from build123d import *

# Parameters (mm, degrees)
SKETCH1_R           = 17.5
BOSS_EXTRUDE1_DEPTH = 150
CUT_EXTRUDE1_START  = 30
CUT_EXTRUDE1_DEPTH  = 30
SKETCH4_W           = 1.6
SKETCH4_H           = 1


with BuildPart() as part:
    # Sketch1 → Boss-Extrude1 (new body)
    with BuildSketch(Plane.XY):
        Circle(SKETCH1_R)
    extrude(amount=BOSS_EXTRUDE1_DEPTH)

    # Sketch3 → Cut-Extrude1 (cut)
    with BuildSketch(Plane.XY.offset(CUT_EXTRUDE1_START)):
        with BuildLine():
            Line((-5, 16.770509831), (-5, 11.770509831))
            Line((-5, 11.770509831), (5, 11.770509831))
            Line((5, 11.770509831), (5, 16.770509831))
            ThreePointArc((5, 16.770509831), (0, 17.5), (-5, 16.770509831))
        make_face()
        with BuildLine():
            Line((16.770509831, 5), (11.770509831, 5))
            Line((11.770509831, 5), (11.770509831, -5))
            Line((11.770509831, -5), (16.770509831, -5))
            ThreePointArc((16.770509831, -5), (17.5, 0), (16.770509831, 5))
        make_face()
    extrude(amount=CUT_EXTRUDE1_DEPTH, mode=Mode.SUBTRACT)

    # Sketch4 → Cut-Revolve1 (revolve, cut)
    with BuildSketch(Plane(origin=(0, 0, 0), x_dir=(0, 0, -1), z_dir=(1, 0, 0)), mode=Mode.PRIVATE) as cut_revolve1_sk:
        with Locations((-29.2, 17)):
            Rectangle(SKETCH4_W, SKETCH4_H)
    revolve(cut_revolve1_sk.sketch.rotate(Axis((0, 0, 0), (0, 0, 1)), 90), axis=Axis((0, 0, 0), (0, 0, 1)), mode=Mode.SUBTRACT)


solid = part.part
Geometry: final body of the model. Coordinates: model frame, mm. A direction names the side the tool comes from. Give positions to 0.01 mm unless a question says otherwise; leave off trailing zeros. Write each loop counter-clockwise with the first axis right and the second up, starting at its lowest first coordinate (ties: lowest second). Pieces come first, ordered by that corner, then holes. Notation, with made-up numbers: (9.25, 30.25) -> (22.25, 30.25) arc R18 ccw to (22.25, 40.25) -> close; hole circle Ø5 at (7.25, -3.75). An arc over 180 degrees is marked (long way). Answer as a JSON object with one key per item and string values.
1. Cut plane D-D on x = 14. Output: boundary loops of the cut face in (y, z), and give its area (3 significant figures).
Ans:
{"outline": "(-10.5, 0) -> (10.5, 0) -> (10.5, 28.4) -> (8.73, 28.4) -> (8.73, 30) -> (10.5, 30) -> (10.5, 150) -> (-10.5, 150) -> (-10.5, 30) -> (-8.73, 30) -> (-8.73, 28.4) -> (-10.5, 28.4) -> close; hole (-5, 30) -> (5, 30) -> (5, 60) -> (-5, 60) -> close", "area": "2,840 mm^2"}
2. Contact query for flat-ended pins moving along their axis: pin 1 (1 mm diameter, centred on y = 3, z = 121, fed in from -X); pin 2 (5.5 mm diameter, centred on y = 14.5, z = 48, fed in from +X); pin 3 (5.5 mm diameter, centred on x = 13, z = 47, fed in from -Y). Output: stop coordinate, or through.
Ans:
{"pin 1": "stops at x = -17.32", "pin 2": "stops at x = 12.97", "pin 3": "stops at y = -14.18"}
3. Cut plane C-C on z = 56.5. Output: boundary loops of the cut face in (x, y).
Ans:
{"outline": "(-5, 11.77) -> (-5, 16.77) arc R17.5 ccw (long way) to (16.77, -5) -> (11.77, -5) -> (11.77, 5) -> (16.77, 5) arc R17.5 ccw to (5, 16.77) -> (5, 11.77) -> close"}
4. Ray query, probe 1 along Z at (x, y) = (-2, 12); probe 2 along Y at (x, z) = (1, 42); probe 3 along Y at (x, z) = (0, 108). Return the intervals inside material, ascending. Write a range as from..to.
Ans:
{"probe 1": "z = 0..30, 60..150", "probe 2": "y = -17.47..11.77", "probe 3": "y = -17.5..17.5"}
5. Access query for faces 1 (the flat face through (14, -5, 45)), 2 (the flat face through (-16, -5, 28.4)), 3 (the flat face through (12, 12, 30)), 4 (the flat face through (5, 14, 45)). Directions: +Z, -Z, +X, -X, +Y, -Y. A direction counts if a zero-diameter tool reaches every point of the face in a straight line with its end or side. Return the directions, or none.
Ans:
{"face 1": "+X", "face 2": "none", "face 3": "+X, +Y", "face 4": "+Y"}
6. Cut plane A-A on x = 0. Output: boundary loops of the cut face in (y, z).
Ans:
{"outline": "(-17.5, 0) -> (17.5, 0) -> (17.5, 28.4) -> (16.5, 28.4) -> (16.5, 30) -> (11.77, 30) -> (11.77, 60) -> (17.5, 60) -> (17.5, 150) -> (-17.5, 150) -> (-17.5, 30) -> (-16.5, 30) -> (-16.5, 28.4) -> (-17.5, 28.4) -> close"}
7. Mould query, pull axis Z, two halves, no side actions, for faces 5 (the cylindrical face through (8.075, -15.526, 89.16)), 6 (the flat face through (0, 0, 150)), 7 (the flat face through (0, 14, 30)). Classes: pulls with the +Z half, pulls with the -Z half, needs draft (parallel to the pull), parting line crosses it, or undercut.
Ans:
{"face 5": "needs draft", "face 6": "pulls with the +Z half", "face 7": "undercut"}
